The model under review builds one solid part; all positions refer to its coordinate system, in mm. A direction names the side the tool comes from. Coordinates: 2 decimals unless noted, no trailing zeros. Loops run counter-clockwise (first coordinate to the right, second up) from the corner with the lowest first, then second, coordinate; pieces in that order, holes last. Notation, with made-up numbers: M -8.5,65.25 L 18.5,65.25 A25 cw 18.5,78.25 Z; hole C 84.5,-6 d9. An arc over 180 degrees is marked long. Return JSON: item names as keys, results as strings.
```python
from build123d import *

# Parameters (mm, degrees)
SKETCH1_W           = 66.04
SKETCH1_H           = 15.24
SKETCH1_R           = 2.99974
SKETCH1_R_2         = 4.7625
BOSS_EXTRUDE1_DEPTH = 19.05
CUT_EXTRUDE2_DEPTH  = 19.05
CUT_EXTRUDE3_START  = -19.05
SKETCH3_R           = 2.00025
CUT_EXTRUDE3_DEPTH  = 19.05
SKETCH4_R           = 1.4986
CUT_EXTRUDE4_DEPTH  = 10.16


with BuildPart() as part:
    # Sketch1 → Boss-Extrude1 (new body)
    with BuildSketch(Plane.XY):
        with Locations((0, -1.27)):
            Rectangle(SKETCH1_W, SKETCH1_H)
        with Locations(Location((-27.02052, 0.35052, 0), (0, 0, 180))):
            Circle(SKETCH1_R, mode=Mode.SUBTRACT)
        with Locations(Location((0, 0, 0), (0, 0, 180))):
            Circle(SKETCH1_R_2, mode=Mode.SUBTRACT)
        with Locations(Location((27.02052, 0.35052, 0), (0, 0, 180))):
            Circle(SKETCH1_R, mode=Mode.SUBTRACT)
    extrude(amount=BOSS_EXTRUDE1_DEPTH)

    # Sketch2 → Cut-Extrude2 (cut)
    with BuildSketch(Plane.ZY.offset(33.02)):
        with BuildLine():
            ThreePointArc((11.52525, -5.76961), (9.525, -3.76936), (7.52475, -5.76961))
            Line((7.52475, -5.76961), (11.52525, -5.76961))
        make_face()
        with BuildLine():
            Line((11.52525, -5.76961), (7.52475, -5.76961))
            ThreePointArc((7.52475, -5.76961), (9.525, -7.76986), (11.52525, -5.76961))
        make_face()
    extrude(amount=-CUT_EXTRUDE2_DEPTH, mode=Mode.SUBTRACT)

    # Sketch3 → Cut-Extrude3 (cut)
    with BuildSketch(Plane(origin=(33.02, 0, 0), x_dir=(0, 0, -1), z_dir=(1, 0, 0)).offset(CUT_EXTRUDE3_START)):
        with Locations(Location((-9.525, -5.76961, 0), (0, 0, 180))):
            Circle(SKETCH3_R)
    extrude(amount=CUT_EXTRUDE3_DEPTH, mode=Mode.SUBTRACT)

    # Sketch4 → Cut-Extrude4 (cut)
    with BuildSketch(Plane(origin=(0, 6.35, 0), x_dir=(1, 0, 0), z_dir=(0, 1, 0))):
        with Locations(Location((9.5885, -5.08, 0), (0, 0, 270))):
            Circle(SKETCH4_R)
        with Locations(Location((9.5885, -13.97, 0), (0, 0, 270))):
            Circle(SKETCH4_R)
        with Locations(Location((-9.5885, -5.08, 0), (0, 0, 270))):
            Circle(SKETCH4_R)
        with Locations(Location((-9.5885, -13.97, 0), (0, 0, 270))):
            Circle(SKETCH4_R)
    extrude(amount=-CUT_EXTRUDE4_DEPTH, mode=Mode.SUBTRACT)


solid = part.part
```
1. The part is to be moulded in two halves that separate along Y. For faces 1 (the face through (-33.02, -1, 9)), 2 (the face through (-24.024, 0.219, 9.392)), 3 (the face through (10, -3.81, 14)), say which applies: released by +Y, released by -Y, zero draft, split by the parting line, or undercut.
Check values:
{"face 1": "zero draft", "face 2": "undercut", "face 3": "released by +Y"}
2. To check wall thickness, follow line 1 (Z direction, x = 9.5, y = -1.25); line 2 (Z direction, x = 9, y = 3.25); line 3 (X direction, y = 2.5, z = 8). State the ranges of each line that lie inside material, in increasing order.
Check values:
{"line 1": "0 to 3.58, 6.58 to 12.47, 15.47 to 19.05", "line 2": "0 to 3.7, 6.46 to 12.59, 15.35 to 19.05", "line 3": "-33.02 to -29.11, -24.93 to -4.05, 4.05 to 24.93, 29.11 to 33.02"}
3. Insertion check: pin 1 Ø3.5 at (x, z) = (-9.59, 5.08) entering from +Y; pin 2 Ø0.9 at (x, z) = (9, 4.5) entering from +Y; pin 3 Ø1.2 at (y, z) = (-6, 8.5) entering from -X; pin 4 Ø2.5 at (y, z) = (-5.77, 9.52) entering from +X. Each pin has a flat end and moves straight along its axis. Give the tip position at first contact, or say it passes through.
Check values:
{"pin 1": "y = 6.35", "pin 2": "y = -3.81", "pin 3": "x = -13.97", "pin 4": "x = 13.97"}
4. Add section A-A on x = 0. Give the boundary of the cut face in (y, z).
Check values:
{"outline": "M -8.89,0 L -4.76,0 L -4.76,19.05 L -8.89,19.05 Z; M 4.76,0 L 6.35,0 L 6.35,19.05 L 4.76,19.05 Z"}
5. Add section B-B on x = 28. State how many separate pieces and enclosed holes the cut face has, plus the area to 3 significant figures.
Check values:
{"separate pieces": "2", "enclosed holes": "1", "area": "170 mm²"}
6. Machinability: for faces 4 (the face through (-13.97, -6, 9)), 5 (the face through (30, 0, 9)), 6 (the face through (23.362, -7.753, 9.265)), 7 (the face through (-10, -3.81, 14)), 8 (the face through (0, -6, 19.05)), which of the approach directions +Z, -Z, +X, -X, +Y, -Y give a long, thin tool a straight path to every point of the face, cutting with its end or side? Answer none if there is none.
Check values:
{"face 4": "-X", "face 5": "+Z, -Z", "face 6": "+X", "face 7": "+Y", "face 8": "+Z, +X, -X, +Y, -Y"}
